from build123d import *

# Parameters (mm, degrees)
CHAMFER_1_SIZE      = 0.5
CUT_EXTRUDE_1_DEPTH = 3


with BuildPart() as part:
    # Эскиз1 → Повернуть1 (revolve)
    with BuildSketch(Plane.XY):
        with BuildLine():
            Line((0, 0), (2.5, 0))
            Line((2.5, 0), (2.5, 15))
            ThreePointArc((2.5, 15), (2.646446609, 15.353553391), (3, 15.5))
            Line((3, 15.5), (4.25, 15.5))
            Line((4.25, 15.5), (4.25, 20))
            ThreePointArc((4.25, 20), (4.103553391, 20.353553391), (3.75, 20.5))
            Line((3.75, 20.5), (0, 20.5))
            Line((0, 20.5), (0, 0))
        make_face()
    revolve(axis=Axis((0, -169.015508263, 0), (0, 1, 0)))

    # Фаска1
    chamfer_1_edges = [part.edges().sort_by_distance(p)[0] for p in [
        (-2.5, 0, 0),
    ]]
    chamfer(chamfer_1_edges, length=CHAMFER_1_SIZE)

    # Эскиз2 → Вырез-Вытянуть1 (cut)
    with BuildSketch(Plane(origin=(0, 20.5, 0), x_dir=(1, 0, 0), z_dir=(0, 1, 0))):
        Polygon((2.309401077, 0), (1.154700538, 2), (-1.154700538, 2), (-2.309401077, 0), (-1.154700538, -2), (1.154700538, -2), align=None)
    extrude(amount=-CUT_EXTRUDE_1_DEPTH, mode=Mode.SUBTRACT)


solid = part.part
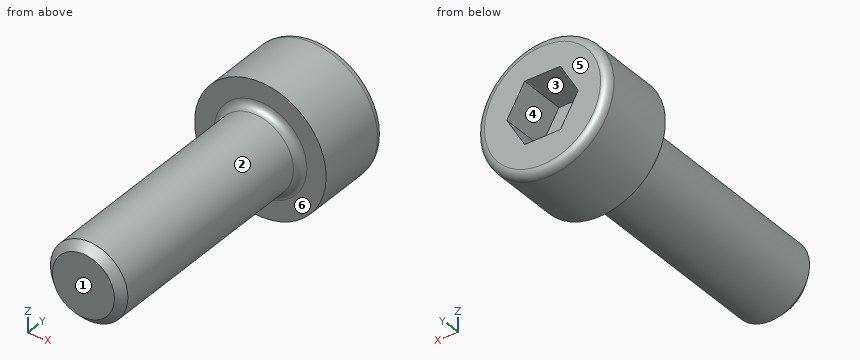
Design review of the part built by this model. Coordinates are the model's own, in mm. Face numbers are marked on the shaded views. A direction names the side the tool comes from. Coordinates: 2 decimals unless noted, no trailing zeros. Order: outer loops, then holes, each group sorted by start corner. A loop starts at its lowest first (then second) coordinate and runs counter-clockwise, first axis right, second up. Notation, with made-up numbers: (14, 84) - (37, 84) arc R29 ccw to (37, 115) - close; hole circle Ø6 at (43, 22). An arc over 180 degrees is marked (long way). Put each result on its own line as item: value.
1) Take a section at A-A, the plane x = 0. Give the boundary of the cut face in (y, z), and give its area (3 significant figures).
Response values:
outline: (0, -2) - (0.5, -2.5) - (15, -2.5) arc R0.5 cw to (15.5, -3) - (15.5, -4.25) - (20, -4.25) arc R0.5 ccw to (20.5, -3.75) - (20.5, -2) - (17.5, -2) - (17.5, 2) - (20.5, 2) - (20.5, 3.75) arc R0.5 ccw to (20, 4.25) - (15.5, 4.25) - (15.5, 3) arc R0.5 cw to (15, 2.5) - (0.5, 2.5) - (0, 2) - close
area: 108 mm²
2) Wall thickness on L1, parallel to X at y = 16, z = 3.75; L2, parallel to Y at x = 1.75, z = -3.25; L3, parallel to Y at x = 1.25, z = -0.5: over which ranges is each line inside the solid? List them lowest first. Write a range as from..to.
Response values:
L1: x = -2..2
L2: y = 15.5..20.5
L3: y = 0..17.5
3) The part is to be moulded in two halves that separate along Z. For the marked faces 1, 2 and 3, say which applies: released by +Z, released by -Z, zero draft, split by the parting line, or undercut.
Response values:
face 1: zero draft
face 2: split by the parting line
face 3: undercut
4) Take a section at B-B, the plane y = 1.75. Give the boundary of the cut face in (x, z).
Response values:
outline: circle Ø5 at (0, 0)
5) Insertion check: P1, Ø1, axis at y = 3, z = -2, coming from the -X side; P2, Ø1.5, axis at y = 11, z = 3, coming from the +X side; P3, Ø2, axis at x = 3, y = 6, coming from the +Z side. Each pin has a flat end and moves straight along its axis. Give the tip position at first contact, or say it passes through.
Response values:
P1: stops at x = -2
P2: stops at x = 1.09
P3: stops at z = 1.5
6) Tool access review of the marked faces 4, 5 and 6: name each direction out of +Z, -Z, +X, -X, +Y, -Y from which nothing blocks a thin tool from reaching the whole face with its end or side.
Response values:
face 4: +Y
face 5: +Z, -Z, +X, -X, +Y
face 6: -Y
